Check sheet for the modelled part. Datum: model origin and axes. Units: mm. A direction names the side the tool comes from. Round coordinates to 2 decimals unless told otherwise and drop trailing zeros. One line per item, written item: value.
from build123d import *

# Parameters (mm, degrees)
BOSS_EXTRUDE1_DEPTH      = 6.35
BOSS_EXTRUDE1_DEPTH_BACK = 6.35
SKETCH2_W                = 292.995908675
SKETCH2_H                = 3.175
CUT_EXTRUDE1_DEPTH       = 38.1
SKETCH3_W                = 146.05
SKETCH3_H                = 3.175
CUT_EXTRUDE2_DEPTH       = 38.1
CUT_EXTRUDE3_DEPTH       = 3.175
CUT_EXTRUDE4_DEPTH       = 3.175
CUT_EXTRUDE5_DEPTH       = 157.099
CUT_EXTRUDE6_DEPTH       = 339.217
CUT_EXTRUDE6_DEPTH_BACK  = 157.099
SKETCH9_W                = 50.8
SKETCH9_H                = 19.05
CUT_EXTRUDE7_DEPTH       = 21.59


with BuildPart() as part:
    # Sketch1 → Boss-Extrude1 (new, two sides: drawn at the far end of the back side and taken through both)
    with BuildSketch(Plane(origin=(0, 0, 0), x_dir=(1, 0, 0), z_dir=(0, 1, 0)).offset(-BOSS_EXTRUDE1_DEPTH_BACK)):
        Polygon((-406.4, 0), (0, 0), (0, 146.05), (-152.4, 146.05), align=None)
    extrude(amount=BOSS_EXTRUDE1_DEPTH + BOSS_EXTRUDE1_DEPTH_BACK)

    # Sketch2 → Cut-Extrude1 (cut)
    with BuildSketch(Plane(origin=(-100.979614843, 0, -175.616721465), x_dir=(-0.8669063030575352, 0, 0.49847112425808277), z_dir=(-0.4984711242580827, 0, -0.8669063030575351))):
        with Locations((205.812767226, 4.7625)):
            Rectangle(SKETCH2_W, SKETCH2_H)
        with Locations((205.812767226, -4.7625)):
            Rectangle(SKETCH2_W, SKETCH2_H)
    extrude(amount=-CUT_EXTRUDE1_DEPTH, mode=Mode.SUBTRACT)

    # Sketch3 → Cut-Extrude2 (cut)
    with BuildSketch(Plane(origin=(0, 0, 0), x_dir=(0, 0, -1), z_dir=(1, 0, 0))):
        with Locations((73.025, 4.7625)):
            Rectangle(SKETCH3_W, SKETCH3_H)
        with Locations((73.025, -4.7625)):
            Rectangle(SKETCH3_W, SKETCH3_H)
    extrude(amount=-CUT_EXTRUDE2_DEPTH, mode=Mode.SUBTRACT)

    # Sketch4 → Cut-Extrude3 (cut)
    with BuildSketch(Plane(origin=(0, 6.35, 0), x_dir=(1, 0, 0), z_dir=(0, 1, 0))):
        Polygon((-133.408250166, 113.020869854), (-75.966284694, 146.05), (-152.4, 146.05), align=None)
    extrude(amount=-CUT_EXTRUDE3_DEPTH, mode=Mode.SUBTRACT)

    # Sketch5 → Cut-Extrude4 (cut)
    with BuildSketch(Plane.XZ.offset(6.35)):
        Polygon((-133.408250166, -113.020869854), (-75.966284694, -146.05), (-152.4, -146.05), align=None)
    extrude(amount=-CUT_EXTRUDE4_DEPTH, mode=Mode.SUBTRACT)

    # Sketch6 → Cut-Extrude5 (cut)
    with BuildSketch(Plane(origin=(0, 0, -146.05), x_dir=(-1, 0, 0), z_dir=(0, 0, -1))):
        Polygon((38.1, -3.175), (43.18, -3.175), (43.18, -6.35), (38.1, -6.35), (0, -6.35), (0, 6.35), (38.1, 6.35), (43.18, 6.35), (43.18, 3.175), (38.1, 3.175), (38.1, 1.5875), (35.56, 1.5875), (35.56, -1.5875), (38.1, -1.5875), align=None)
    extrude(amount=-CUT_EXTRUDE5_DEPTH, mode=Mode.SUBTRACT)

    # Sketch8 → Cut-Extrude6 (cut, two sides: drawn at the far end of the back side and taken through both)
    with BuildSketch(Plane(origin=(-51.420385157, 0, 29.566721465), x_dir=(0.49847112425808243, 0, 0.8669063030575355), z_dir=(-0.8669063030575355, 0, 0.49847112425808243)).offset(-CUT_EXTRUDE6_DEPTH_BACK)):
        Polygon((-164.478664898, 3.175), (-159.398664898, 3.175), (-159.398664898, 6.35), (-164.478664898, 6.35), (-202.578664898, 6.35), (-202.578664898, -6.35), (-164.478664898, -6.35), (-159.398664898, -6.35), (-159.398664898, -3.175), (-164.478664898, -3.175), (-164.478664898, -1.5875), (-167.018664898, -1.5875), (-167.018664898, 1.5875), (-164.478664898, 1.5875), align=None)
    extrude(amount=CUT_EXTRUDE6_DEPTH + CUT_EXTRUDE6_DEPTH_BACK, mode=Mode.SUBTRACT)

    # Sketch9 → Cut-Extrude7 (cut)
    with BuildSketch(Plane(origin=(0, 6.35, 0), x_dir=(1, 0, 0), z_dir=(0, 1, 0))):
        with Locations((-25.4, 136.525)):
            Rectangle(SKETCH9_W, SKETCH9_H)
    extrude(amount=-CUT_EXTRUDE7_DEPTH, mode=Mode.SUBTRACT)


solid = part.part
Q1. Depth check by flat-ended pin: P1, Ø3.5, axis at y = -4.5, z = -60.5, coming from the +X side; P2, Ø4, axis at x = -186.5, y = 0.5, coming from the -Z side; P3, Ø1, axis at y = 1.5, z = -15.5, coming from the -X side. Enter the tip coordinate at first touch or a pass-through.
Completed:
P1: x = -38.1
P2: z = -86.57
P3: x = -308.97
Q2. Scan lines: line 1 (X direction, y = 3.25, z = -7.5); line 2 (X direction, y = -4.5, z = -105.5); line 3 (Z direction, x = -71, y = 3.25). Record each from-to range of solid material in increasing order. Write a range as [from, to].
Completed:
line 1: [-306.73, -43.18]
line 2: [-136.3, -43.18]
line 3: [-143.05, 0]
Q3. Access from +Z, -Z, +X, -X, +Y, -Y to the whole of each face (thin tool, end or side, straight path). Record for faces 1 (the flat face through (-201.188, 2.37, -74.047)), 2 (the flat face through (-50.8, 0, -136)), 3 (the flat face through (-41, -3.175, -64)), 4 (the flat face through (-196, -3.175, -74)), 5 (the flat face through (-41, 3.175, -64)).
Completed:
face 1: -Z, -X, +Y
face 2: -Z, +X, +Y, -Y
face 3: +Z, -Z, +X, -Y
face 4: -Z, -X, -Y
face 5: +Z, -Z, +X, +Y
